Part model, mm, in its own coordinate system. Face numbers are marked on the shaded views. A direction names the side the tool comes from. Give positions to 0.01 mm unless a question says otherwise; leave off trailing zeros. Write each loop counter-clockwise with the first axis right and the second up, starting at its lowest first coordinate (ties: lowest second). Pieces come first, ordered by that corner, then holes.
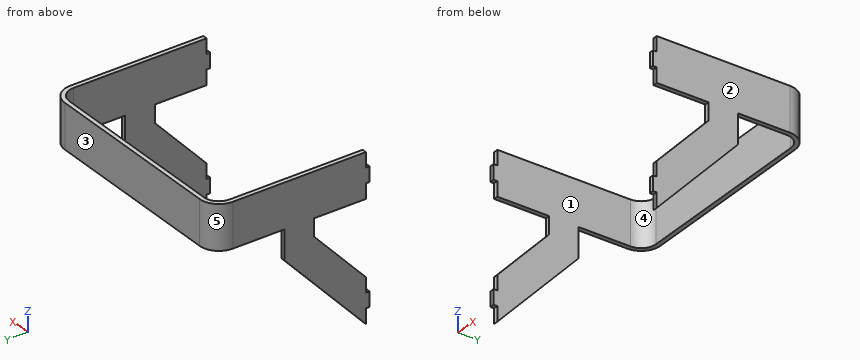
```python
from build123d import *

# Parameters (mm, degrees)
BOSS_EXTRUDE1_DEPTH = 30
BOSS_EXTRUDE2_START = 73
BOSS_EXTRUDE2_DEPTH = 3
SKETCH3_W           = 3
SKETCH3_H           = 10
BOSS_EXTRUDE3_DEPTH = 2.5


with BuildPart() as part:
    # Sketch1 → Boss-Extrude1 (new body)
    with BuildSketch(Plane.XY):
        with BuildLine():
            Line((-73, 0), (-73, 90))
            ThreePointArc((-73, 90), (-70.071067812, 97.071067812), (-63, 100))
            Line((-63, 100), (63, 100))
            ThreePointArc((63, 100), (70.071067812, 97.071067812), (73, 90))
            Line((73, 90), (73, 0))
            Line((73, 0), (76, 0))
            Line((76, 0), (76, 90))
            ThreePointArc((76, 90), (72.192388155, 99.192388155), (63, 103))
            Line((63, 103), (-63, 103))
            ThreePointArc((-63, 103), (-72.192388155, 99.192388155), (-76, 90))
            Line((-76, 90), (-76, 0))
            Line((-76, 0), (-73, 0))
        make_face()
    extrude(amount=BOSS_EXTRUDE1_DEPTH)

    # Sketch2 → Boss-Extrude2 (add)
    with BuildSketch(Plane(origin=(0, 0, 0), x_dir=(0, 0, -1), z_dir=(1, 0, 0)).offset(BOSS_EXTRUDE2_START)):
        Polygon((0, 55), (20, 55), (80, 0), (50, 0), (11.818181818, 35), (0, 35), align=None)
    boss_extrude2 = extrude(amount=BOSS_EXTRUDE2_DEPTH)

    # Mirror1: Boss-Extrude2 across plane
    add(boss_extrude2.mirror(Plane(origin=(0, 0, 0), x_dir=(0, 0, 1), z_dir=(1, 0, 0))))

    # Sketch3 → Boss-Extrude3 (add)
    with BuildSketch(Plane.XZ):
        with Locations((-74.5, 15)):
            Rectangle(SKETCH3_W, SKETCH3_H)
        with Locations((-74.5, -65)):
            Rectangle(SKETCH3_W, SKETCH3_H)
        with Locations((74.5, -65)):
            Rectangle(SKETCH3_W, SKETCH3_H)
        with Locations((74.5, 15)):
            Rectangle(SKETCH3_W, SKETCH3_H)
    extrude(amount=BOSS_EXTRUDE3_DEPTH)


solid = part.part
```
1) Saw through at A-A, the plane z = -4. Write the cut outline in (x, y), then the cut area to 3 significant figures.
Answers follow:
outline: (-76, 35) - (-73, 35) - (-73, 55) - (-76, 55) - close; (73, 35) - (76, 35) - (76, 55) - (73, 55) - close
area: 120 mm2
2) Wall check: L1, parallel to X at y = 21, z = -33.5; L2, parallel to Y at x = -35.5, z = 23. Give the ranges that are in metal, low to high.
Answers follow:
L1: x = -76 to -73, 73 to 76
L2: y = 100 to 103
3) Pin check, flat tips, straight feed: pin 1 Ø1.5 at (x, z) = (75, 2.5) entering from -Y; pin 2 Ø15 at (x, z) = (3, 15) entering from -Y; pin 3 Ø0.9 at (x, z) = (-74, -8.5) entering from -Y. Stop position of each tip, or through.
Answers follow:
pin 1: stops at y = 0
pin 2: stops at y = 100
pin 3: stops at y = 35
4) Two-plate mould, pull along X, no slides. Class the marked faces 1, 2 and 3: +X half, -X half, draft (parallel to the pull), parting line (faces both ways), or undercut.
Answers follow:
face 1: undercut
face 2: +X half
face 3: draft
5) 3-axis set-ups, long thin cutter, end or side, ignore diameter. For the marked faces 4 and 5: which of +Z, -Z, +X, -X, +Y, -Y reach the whole face in a straight line?
Answers follow:
face 4: +Z, -Z, -Y
face 5: +Z, -Z, -X, +Y
6) Saw through at D-D, the plane x = 42. Write the cut outline in (y, z), then the cut area to 3 significant figures.
Answers follow:
outline: (100, 0) - (103, 0) - (103, 30) - (100, 30) - close
area: 90.0 mm2
7) Saw through at B-B, the plane y = 63.5. Write the cut outline in (x, z).
Answers follow:
outline: (-76, 0) - (-73, 0) - (-73, 30) - (-76, 30) - close; (73, 0) - (76, 0) - (76, 30) - (73, 30) - close
8) Saw through at C-C, the plane y = 20.5. Write the cut outline in (x, z).
Answers follow:
outline: (-76, -57.64) - (-73, -57.64) - (-73, -27.64) - (-76, -27.64) - close; (-76, 0) - (-73, 0) - (-73, 30) - (-76, 30) - close; (73, -57.64) - (76, -57.64) - (76, -27.64) - (73, -27.64) - close; (73, 0) - (76, 0) - (76, 30) - (73, 30) - close
